Answer from the drawing. Dimensions are ordinates in mm from the lowest x, y and z of the part. A direction names the side the tool comes from. Round coordinates to 2 decimals unless told otherwise and drop trailing zeros. Write each loop counter-clockwise with the first axis right and the second up, starting at its lowest first coordinate (ties: lowest second). Pieces come first, ordered by that corner, then holes. Notation, with made-up numbers: (81, 0) -> (138, 0) arc R37 cw to (138, 37) -> close; hole circle Ø7 at (79, 21). An arc over 180 degrees is marked (long way). Return JSON: item names as keys, results as strings. Group by question number.
(1) A cutting plane is placed at B-B on z = 10. Give the vertices of the cut face in (x, y).
(2) For the marked faces 4 and 5, determine the directions among +Z, -Z, +X, -X, +Y, -Y from which every point of the face is accessible in a straight line to the end or side of a thin tool.
(3) A cutting plane is placed at A-A on y = 10. Give the vertices of the cut face in (x, z).
(4) A cutting plane is placed at D-D on y = 16.75. Give the vertices of the cut face in (x, z), then the cut area to 3 significant figures.
(5) A cutting plane is placed at C-C on x = 34. Give the vertices of the cut face in (y, z).
(6) Given pin 1 (1.5 mm diameter, centred on x = 32, y = 6, fed in from -Z); pin 2 (8 mm diameter, centred on x = 22, z = 10.5, fed in from +Y); pin 3 (5.5 mm diameter, centred on x = 34, y = 10, fed in from -Z), each flat-ended and moving along its own axis, determine where each tip first touches the part or whether it passes through.
(7) The mould has two halves that part along X. Classify the marked faces 1, 2 and 3: released by +X, released by -X, zero draft, split by the parting line, or undercut.
(8) Straight lines are drawn through the part: line 1 (Z direction, x = 14, y = 1.5); line 2 (X direction, y = 7, z = 7); line 3 (Y direction, x = 4.5, z = 2). For each, find the intervals that lie inside material, in ascending order.
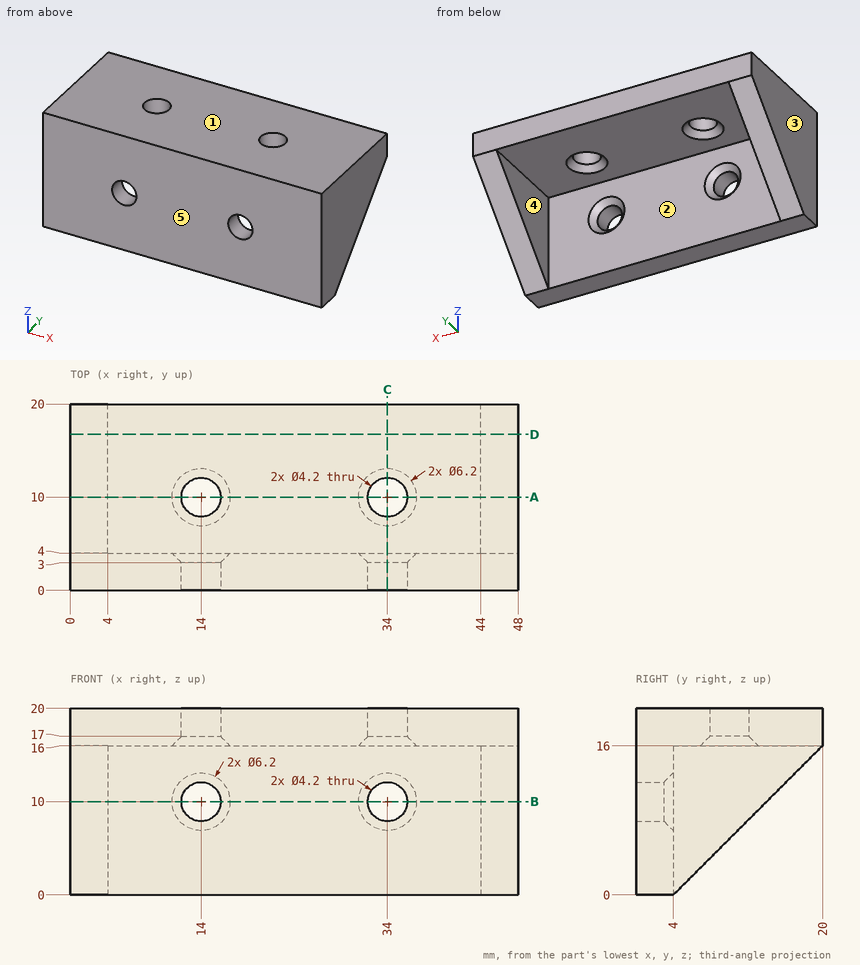
Checks:
{
 "1": {"outline": "(0, 0) -> (11.9, 0) -> (11.9, 3) -> (10.9, 4) -> (4, 4) -> (4, 14) -> (0, 14) -> close; (16.1, 0) -> (31.9, 0) -> (31.9, 3) -> (30.9, 4) -> (17.1, 4) -> (16.1, 3) -> close; (36.1, 0) -> (48, 0) -> (48, 14) -> (44, 14) -> (44, 4) -> (37.1, 4) -> (36.1, 3) -> close"},
 "2": {"face 4": "-Z, +Y", "face 5": "+Z, -Z, +X, -X, -Y"},
 "3": {"outline": "(0, 6) -> (4, 6) -> (4, 16) -> (10.9, 16) -> (11.9, 17) -> (11.9, 20) -> (0, 20) -> close; (16.1, 17) -> (17.1, 16) -> (30.9, 16) -> (31.9, 17) -> (31.9, 20) -> (16.1, 20) -> close; (36.1, 17) -> (37.1, 16) -> (44, 16) -> (44, 6) -> (48, 6) -> (48, 20) -> (36.1, 20) -> close"},
 "4": {"outline": "(0, 12.75) -> (4, 12.75) -> (4, 16) -> (44, 16) -> (44, 12.75) -> (48, 12.75) -> (48, 20) -> (0, 20) -> close", "area": "218 mm^2"},
 "5": {"outline": "(0, 0) -> (4, 0) -> (4, 6.9) -> (3, 7.9) -> (0, 7.9) -> close; (0, 12.1) -> (3, 12.1) -> (4, 13.1) -> (4, 16) -> (6.9, 16) -> (7.9, 17) -> (7.9, 20) -> (0, 20) -> close; (12.1, 17) -> (13.1, 16) -> (20, 16) -> (20, 20) -> (12.1, 20) -> close"},
 "6": {"pin 1": "stops at z = 16", "pin 2": "stops at y = 4", "pin 3": "stops at z = 16.35"},
 "7": {"face 1": "zero draft", "face 2": "undercut", "face 3": "released by -X"},
 "8": {"line 1": "z = 0 to 7.9, 12.1 to 20", "line 2": "x = 0 to 4, 44 to 48", "line 3": "y = 0 to 4"}
}
